Geometry: see drawing. Coordinates: mm, zero at the bounding-box minimum. Give positions to 0.01 mm unless a question says otherwise; leave off trailing zeros. Loops run counter-clockwise (first coordinate to the right, second up) from the corner with the lowest first, then second, coordinate; pieces in that order, holes last. Notation, with made-up numbers: M -11.5,7.25 L -1.5,7.25 A18 ccw -1.5,17.25 Z; hole C -35,63.5 d4. An arc over 180 degrees is marked long. Answer in a Markdown table with one row per item.
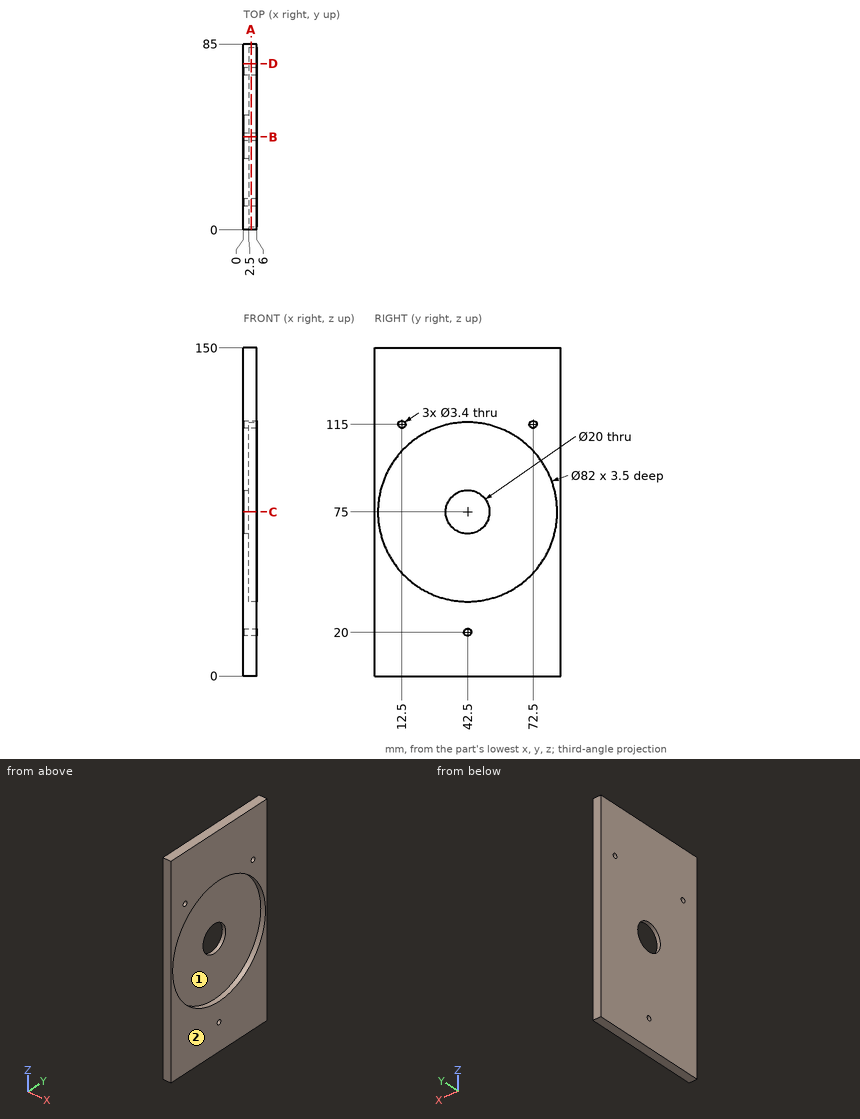
1) Section C-C, the plane z = 75. Return loops of the section in (x, y), then the cut area to 3 significant figures.
Reply:
| item | result |
|---|---|
| outline | M 0,0 L 6,0 L 6,1.5 L 2.5,1.5 L 2.5,32.5 L 0,32.5 Z; M 0,52.5 L 2.5,52.5 L 2.5,83.5 L 6,83.5 L 6,85 L 0,85 Z |
| area | 173 mm² |
2) Material intervals for L1, parallel to Y at x = 1, z = 75; L2, parallel to Y at x = 5, z = 49; L3, parallel to Z at x = 5.25, y = 72, sorted ascending.
Reply:
| item | result |
|---|---|
| L1 | y = 0 to 32.5, 52.5 to 85 |
| L2 | y = 0 to 10.8, 74.2 to 85 |
| L3 | z = 0 to 46.53, 103.47 to 113.38, 116.62 to 150 |
3) Section B-B, the plane y = 42.5. Return loops of the section in (x, z), then the cut area to 3 significant figures.
Reply:
| item | result |
|---|---|
| outline | M 0,0 L 6,0 L 6,18.3 L 0,18.3 Z; M 0,21.7 L 6,21.7 L 6,34 L 2.5,34 L 2.5,65 L 0,65 Z; M 0,85 L 2.5,85 L 2.5,116 L 6,116 L 6,150 L 0,150 Z |
| area | 543 mm² |
4) Pin query (flat end, axial travel): pin 1 Ø4 at (y, z) = (72.5, 115) entering from -X. Return the tip coordinate at first contact, or that it passes through.
Reply:
| item | result |
|---|---|
| pin 1 | stops at x = 0 |
5) Section A-A, the plane x = 3.5. Return loops of the section in (y, z).
Reply:
| item | result |
|---|---|
| outline | M 0,0 L 85,0 L 85,150 L 0,150 Z; hole C 42.5,75 d82; hole C 12.5,115 d3.4; hole C 42.5,20 d3.4; hole C 72.5,115 d3.4 |
6) Pull-direction query (Y, two-part tool) for the marked faces 1 and 2; classes: released by +Y, released by -Y, zero draft, split by the parting line, or undercut.
Reply:
| item | result |
|---|---|
| face 1 | undercut |
| face 2 | zero draft |
7) Section D-D, the plane y = 76. Return loops of the section in (x, z), then the cut area to 3 significant figures.
Reply:
| item | result |
|---|---|
| outline | M 0,0 L 6,0 L 6,51.36 L 2.5,51.36 L 2.5,98.64 L 6,98.64 L 6,150 L 0,150 Z |
| area | 735 mm² |
